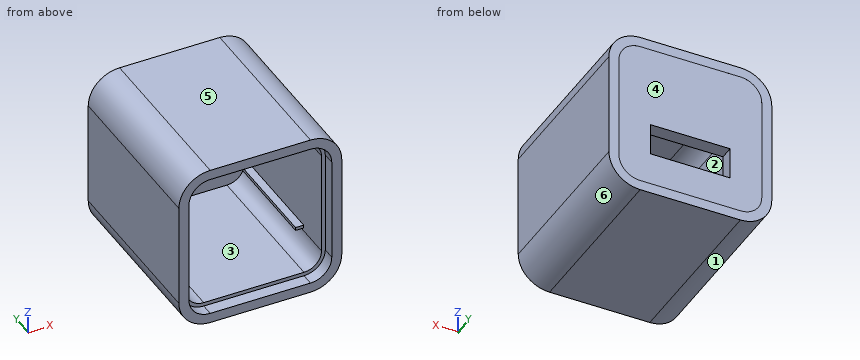
```python
from build123d import *

# Parameters (mm, degrees)
RESSALTO_EXTRUS_O1_DEPTH = 28
CASCA1_T                 = -2.2
ESBO_O2_W                = 12.7
ESBO_O2_H                = 5.1
CORTE_EXTRUS_O1_DEPTH    = 5
CORTE_EXTRUS_O2_DEPTH    = 0.001
CORTE_EXTRUS_O3_START    = -2
CORTE_EXTRUS_O3_DEPTH    = 2
ESBO_O5_W                = 1.3
ESBO_O5_H                = 0.5
RESSALTO_EXTRUS_O2_DEPTH = 18.3


with BuildPart() as part:
    # Esboço1 → Ressalto-extrusão1 (new body)
    with BuildSketch(Plane(origin=(0, 0, 0), x_dir=(1, 0, 0), z_dir=(0, 1, 0))):
        with BuildLine():
            Line((-8, -13.3), (8, -13.3))
            ThreePointArc((8, -13.3), (11.535533906, -11.835533906), (13, -8.3))
            Line((13, -8.3), (13, 8.3))
            ThreePointArc((13, 8.3), (11.535533906, 11.835533906), (8, 13.3))
            Line((8, 13.3), (-8, 13.3))
            ThreePointArc((-8, 13.3), (-11.535533906, 11.835533906), (-13, 8.3))
            Line((-13, 8.3), (-13, -8.3))
            ThreePointArc((-13, -8.3), (-11.535533906, -11.835533906), (-8, -13.3))
        make_face()
    extrude(amount=RESSALTO_EXTRUS_O1_DEPTH)

    # Casca1
    casca1_openings = [part.faces().sort_by_distance(p)[0] for p in [
        (0, 0, 0),
    ]]
    offset(amount=CASCA1_T, openings=casca1_openings, kind=Kind.INTERSECTION)

    # Esboço2 → Corte-extrusão1 (cut)
    with BuildSketch(Plane(origin=(0, 28, 0), x_dir=(-1, 0, 0), z_dir=(0, 1, 0))):
        with Locations((0, -3.95)):
            Rectangle(ESBO_O2_W, ESBO_O2_H)
    extrude(amount=-CORTE_EXTRUS_O1_DEPTH, mode=Mode.SUBTRACT)

    # Esboço3 → Corte-extrusão2 (cut)
    with BuildSketch(Plane(origin=(0, 28, 0), x_dir=(1, 0, 0), z_dir=(0, 1, 0))):
        with BuildLine():
            Line((-8, -11.7), (8, -11.7))
            ThreePointArc((8, -11.7), (10.404163056, -10.704163056), (11.4, -8.3))
            Line((11.4, -8.3), (11.4, 8.3))
            ThreePointArc((11.4, 8.3), (10.404163056, 10.704163056), (8, 11.7))
            Line((8, 11.7), (-8, 11.7))
            ThreePointArc((-8, 11.7), (-10.404163056, 10.704163056), (-11.4, 8.3))
            Line((-11.4, 8.3), (-11.4, -8.3))
            ThreePointArc((-11.4, -8.3), (-10.404163056, -10.704163056), (-8, -11.7))
        make_face()
    extrude(amount=-CORTE_EXTRUS_O2_DEPTH, mode=Mode.SUBTRACT)

    # Esboço4 → Corte-extrusão3 (cut)
    with BuildSketch(Plane.XZ.offset(CORTE_EXTRUS_O3_START)):
        with BuildLine():
            Line((-8, -11.7), (8, -11.7))
            ThreePointArc((8, -11.7), (10.404163056, -10.704163056), (11.4, -8.3))
            Line((11.4, -8.3), (11.4, 8.3))
            ThreePointArc((11.4, 8.3), (10.404163056, 10.704163056), (8, 11.7))
            Line((8, 11.7), (-8, 11.7))
            ThreePointArc((-8, 11.7), (-10.404163056, 10.704163056), (-11.4, 8.3))
            Line((-11.4, 8.3), (-11.4, -8.3))
            ThreePointArc((-11.4, -8.3), (-10.404163056, -10.704163056), (-8, -11.7))
        make_face()
    extrude(amount=CORTE_EXTRUS_O3_DEPTH, mode=Mode.SUBTRACT)

    # Esboço5 → Ressalto-extrusão2 (add)
    with BuildSketch(Plane.XZ.offset(-25.8)):
        with Locations((10.15, -7.55)):
            Rectangle(ESBO_O5_W, ESBO_O5_H)
    ressalto_extrus_o2 = extrude(amount=RESSALTO_EXTRUS_O2_DEPTH)

    # Espelhar1: Ressalto-extrusão2 across plane
    add(ressalto_extrus_o2.mirror(Plane(origin=(0, 0, 0), x_dir=(0, 0, 1), z_dir=(1, 0, 0))))


solid = part.part
```
CAD build for the part. Positions are in the model's coordinates, mm. Face numbers are marked on the shaded views. A direction names the side the tool comes from. Round coordinates to 2 decimals unless told otherwise and drop trailing zeros. Order: outer loops, then holes, each group sorted by start corner. A loop starts at its lowest first (then second) coordinate and runs counter-clockwise, first axis right, second up.
Q1. Slice it at A-A (y = 26.5). Write the cut outline in (x, z), and give its area (3 significant figures).
Q2. Wall check: L1, parallel to Z at x = -1, y = 1.75; L2, parallel to Z at x = 3.75, y = 14.75; L3, parallel to X at y = 19, z = -5.5. Give the ranges that are in metal, low to high.
Q3. Which spindle directions (+Z, -Z, +X, -X, +Y, -Y) get a long thin tool onto all of the face, cutting with end or side? Do the marked faces 1 and 2. Say none if no direction does.
Q4. Drop flat-ended pins along their axis: pin 1 (0.7 mm diameter, centred on x = -10.5, y = 20.5, fed in from +Z); pin 2 (1.4 mm diameter, centred on x = -10.5, y = 14, fed in from -Z); pin 3 (2 mm diameter, centred on x = 5, z = -7.5, fed in from -Y); pin 4 (1.5 mm diameter, centred on x = -8.5, y = 11.5, fed in from +Z). Give the stop position or say it passes through.
Q5. Two-plate mould, pull along Z, no slides. Class the marked faces 3, 4, 5 and 6: pulls with the +Z half, pulls with the -Z half, needs draft (parallel to the pull), parting line crosses it, or undercut.
Results below:
1. outline: (-13, -8.3) arc R5 ccw to (-8, -13.3) - (8, -13.3) arc R5 ccw to (13, -8.3) - (13, 8.3) arc R5 ccw to (8, 13.3) - (-8, 13.3) arc R5 ccw to (-13, 8.3) - close; hole (-6.35, -6.5) - (6.35, -6.5) - (6.35, -1.4) - (-6.35, -1.4) - close
1. area: 605 mm2
2. L1: z = -13.3 to -11.7, 11.7 to 13.3
2. L2: z = -13.3 to -11.1, 11.1 to 13.3
2. L3: x = -13 to -10.8, 10.8 to 13
3. face 1: -Z, -X, +Y, -Y
3. face 2: -Y
4. pin 1: stops at z = 12.81
4. pin 2: stops at z = -12.96
4. pin 3: stops at y = 25.8
4. pin 4: stops at z = 13.3
5. face 3: undercut
5. face 4: needs draft
5. face 5: pulls with the +Z half
5. face 6: pulls with the -Z half
